The model under review builds one solid part; all positions refer to its coordinate system, in mm. A direction names the side the tool comes from. Give positions to 0.01 mm unless a question says otherwise; leave off trailing zeros. Order: outer loops, then holes, each group sorted by start corner. A loop starts at its lowest first (then second) coordinate and runs counter-clockwise, first axis right, second up. Notation, with made-up numbers: (32.25, -22.5) - (52.25, -22.5) arc R6 cw to (52.25, -13.5) - close; hole circle Ø5 at (32, -29). An arc over 180 degrees is marked (long way). Use CSV: the item, a comma, the result in double quotes.
```python
from build123d import *

# Parameters (mm, degrees)
BOSS_EXTRUDE1_DEPTH = 29.4
BOSS_EXTRUDE2_DEPTH = 21.7


with BuildPart() as part:
    # Sketch1 → Boss-Extrude1 (new, symmetric)
    with BuildSketch(Plane(origin=(0, 0, 0), x_dir=(0, 0, -1), z_dir=(1, 0, 0))):
        Polygon((-16, 6), (16, 6), (16, -6), (7.5, -6), (7.5, 0), (-7.5, 0), (-7.5, -6), (-16, -6), align=None)
    extrude(amount=BOSS_EXTRUDE1_DEPTH, both=True)

    # Sketch2 → Boss-Extrude2 (add, symmetric)
    with BuildSketch(Plane(origin=(0, 0, 0), x_dir=(0, 0, -1), z_dir=(1, 0, 0))):
        Polygon((-16, -6), (-16.5, -6), (-16.5, 6.5), (16.5, 6.5), (16.5, -6), (16, -6), (16, 6), (-16, 6), align=None)
    extrude(amount=BOSS_EXTRUDE2_DEPTH, both=True)


solid = part.part
```
Item 1: Mouldability with a two-part tool opening along Z and no side actions: class faces 5 (the face through (0, 0, 16.5)), 6 (the face through (-21.7, 6.3, -0.1)), 7 (the face through (0, -3, 7.5)) as pulls with the +Z half, pulls with the -Z half, needs draft (parallel to the pull), parting line crosses it, or undercut.
Results list:
face 5,"pulls with the +Z half"
face 6,"needs draft"
face 7,"undercut"
Item 2: Take a section at C-C, the plane x = 9.5. Give the boundary of the cut face in (y, z).
Results list:
outline,"(-6, -16.5) - (6.5, -16.5) - (6.5, 16.5) - (-6, 16.5) - (-6, 7.5) - (0, 7.5) - (0, -7.5) - (-6, -7.5) - close"
Item 3: Take a section at A-A, the plane y = -2.75. Give the boundary of the cut face in (x, z), and give its area (3 significant figures).
Results list:
outline,"(-29.4, -16) - (-21.7, -16) - (-21.7, -16.5) - (21.7, -16.5) - (21.7, -16) - (29.4, -16) - (29.4, -7.5) - (-29.4, -7.5) - close; (-29.4, 7.5) - (29.4, 7.5) - (29.4, 16) - (21.7, 16) - (21.7, 16.5) - (-21.7, 16.5) - (-21.7, 16) - (-29.4, 16) - close"
area,"1,040 mm2"
Item 4: Clearance check with flat-ended pins moving along their axes: pin 1 (4 mm diameter, centred on y = -1, z = -1, fed in from +X); pin 2 (2.5 mm diameter, centred on x = 27, z = -3, fed in from +Y); pin 3 (2.5 mm diameter, centred on x = -24, y = 2.5, fed in from +Z); pin 4 (10 mm diameter, centred on x = -9.5, z = -0.5, fed in from -Y). State where each tip first meets the part, or that it passes through.
Results list:
pin 1,"stops at x = 29.4"
pin 2,"stops at y = 6"
pin 3,"stops at z = 16"
pin 4,"stops at y = 0"
Item 5: Tool access review of faces 1 (the face through (-25, 0, -16)), 2 (the face through (0, -3, -7.5)), 3 (the face through (26, 6, 0)), 4 (the face through (-25, 0, 16)): name each direction out of +Z, -Z, +X, -X, +Y, -Y from which nothing blocks a thin tool from reaching the whole face with its end or side.
Results list:
face 1,"-Z, -X, +Y, -Y"
face 2,"+X, -X, -Y"
face 3,"+Z, -Z, +X, +Y"
face 4,"+Z, -X, +Y, -Y"
Item 6: Take a section at B-B, the plane z = -0.5. Give the boundary of the cut face in (x, y), and give its area (4 significant figures).
Results list:
outline,"(-29.4, 0) - (29.4, 0) - (29.4, 6) - (21.7, 6) - (21.7, 6.5) - (-21.7, 6.5) - (-21.7, 6) - (-29.4, 6) - close"
area,"374.5 mm2"
Item 7: Wall thickness on L1, parallel to Z at x = -23.5, y = -3.5; L2, parallel to Z at x = 10.5, y = -2.5; L3, parallel to Y at x = -20, z = -4.5: over which ranges is each line inside the solid? List them lowest first.
Results list:
L1,"z = -16 to -7.5, 7.5 to 16"
L2,"z = -16.5 to -7.5, 7.5 to 16.5"
L3,"y = 0 to 6.5"
